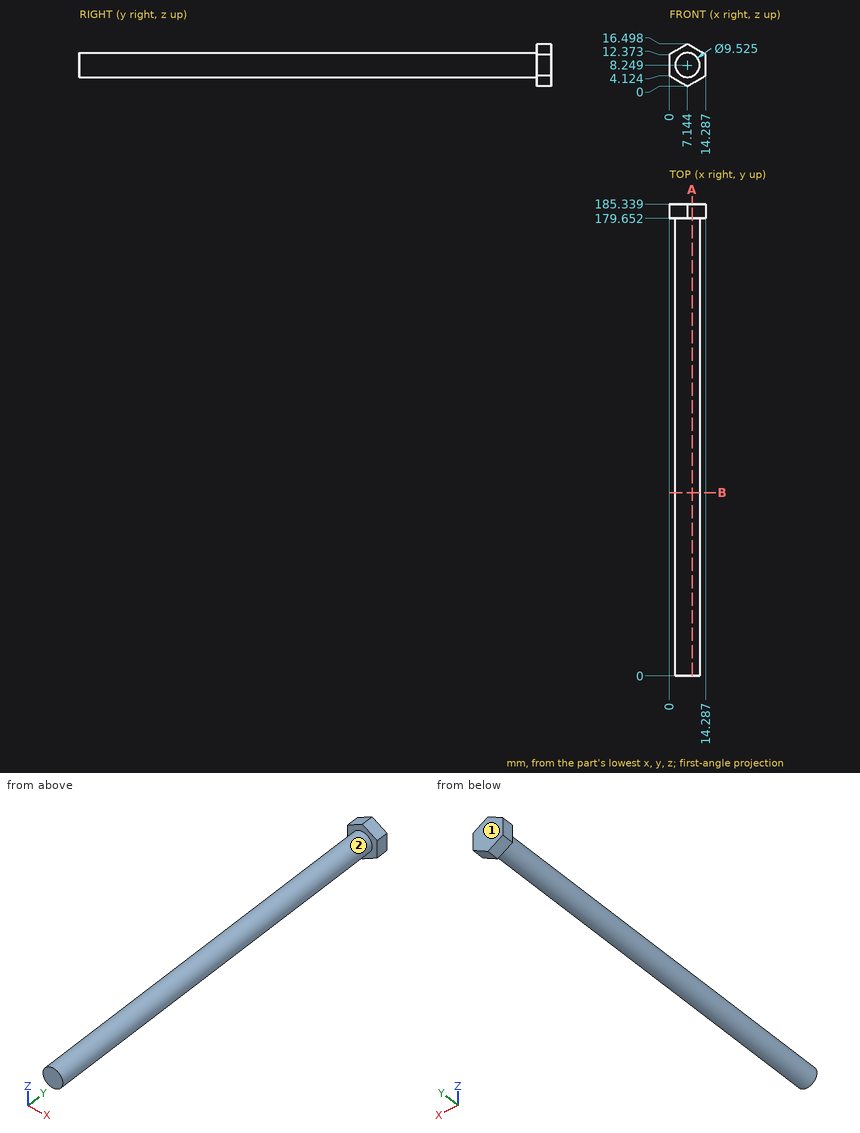
Can you work these out from the drawing? Everything is in mm from the part's minimum corner. A direction names the side the tool comes from. Give positions to 0.01 mm unless a question says otherwise; leave off trailing zeros. Loops run counter-clockwise (first coordinate to the right, second up) from the corner with the lowest first, then second, coordinate; pieces in that order, holes last. Notation, with made-up numbers: (18, 61.5) - (57, 61.5) arc R24 cw to (57, 74.5) - close; hole circle Ø9 at (5, 56.25). An arc over 180 degrees is marked (long way). Answer as a JSON object with one key per item and string values.
Q1. Imagine slicing it at A-A on x = 9. Write out the boundary of the cut face in (y, z) (1 decimal), plus the area to 3 significant figures.
Geometry says:
{"outline": "(0, 3.9) - (179.7, 3.9) - (179.7, 1.1) - (185.3, 1.1) - (185.3, 15.4) - (179.7, 15.4) - (179.7, 12.6) - (0, 12.6) - close", "area": "1,660 mm²"}
Q2. Will these pins go through, and if not, where does the flat tip stop? P1, Ø4, axis at x = 3.5, y = 134.5, coming from the -Z side; P2, Ø5, axis at x = 4.5, y = 116, coming from the -Z side; P3, Ø1, axis at y = 157.5, z = 10.5, coming from the +X side.
Geometry says:
{"P1": "z = 3.78", "P2": "z = 3.49", "P3": "x = 11.57"}
Q3. If I drill on L1, parallel to Y at x = 10.5, z = 3; L2, parallel to Z at x = 7, y = 34.5; L3, parallel to X at y = 77, z = 8.5, over which ranges is the centre line in solid material (lowest first)?
Geometry says:
{"L1": "179.65 to 185.34", "L2": "3.49 to 13.01", "L3": "2.39 to 11.9"}
Q4. Imagine slicing it at B-B on y = 72. Write out the boundary of the cut face in (x, z) (1 decimal).
Geometry says:
{"outline": "circle Ø9.5 at (7.1, 8.2)"}
Q5. Which directions (+Z, -Z, +X, -X, +Y, -Y) give clear straight access to the entire face, cutting with the end or side of a thin tool? Please do the marked faces 1 and 2.
Geometry says:
{"face 1": "+Z, -Z, +X, -X, +Y", "face 2": "-Y"}
